Could you check a few things on this model? Use its own coordinates, in mm. Face numbers are marked on the shaded views. A direction names the side the tool comes from. Give positions to 0.01 mm unless a question says otherwise; leave off trailing zeros. Write each loop counter-clockwise with the first axis right and the second up, starting at its lowest first coordinate (ties: lowest second). Pieces come first, ordered by that corner, then holes. Notation, with made-up numbers: M 68,-15.5 L 72,-15.5 A23 ccw 72,16.5 Z; hole C -37.75,-9 d9. An arc over 180 degrees is marked long. Use one line per item in the form item = value.
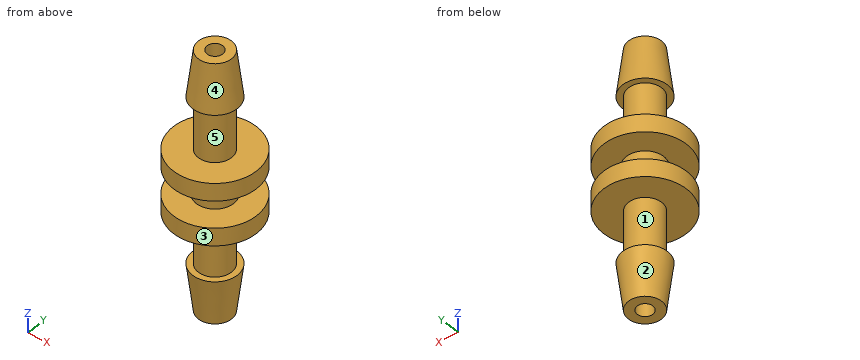
from build123d import *

# Parameters (mm, degrees)
SKETCH1_R           = 1.8
SKETCH1_R_2         = 0.75
BOSS_EXTRUDE1_DEPTH = 1.3
SKETCH2_R           = 4
SKETCH2_R_2         = 0.75
BOSS_EXTRUDE2_DEPTH = 1.7
SKETCH3_R           = 1.6
SKETCH3_R_2         = 0.75
BOSS_EXTRUDE3_DEPTH = 5


with BuildPart() as part:
    # Sketch1 → Boss-Extrude1 (new body)
    with BuildSketch(Plane.XY):
        Circle(SKETCH1_R)
        Circle(SKETCH1_R_2, mode=Mode.SUBTRACT)
    boss_extrude1 = extrude(amount=BOSS_EXTRUDE1_DEPTH)

    # Sketch2 → Boss-Extrude2 (add)
    with BuildSketch(Plane.XY.offset(1.3)):
        Circle(SKETCH2_R)
        Circle(SKETCH2_R_2, mode=Mode.SUBTRACT)
    boss_extrude2 = extrude(amount=BOSS_EXTRUDE2_DEPTH)

    # Sketch3 → Boss-Extrude3 (add)
    with BuildSketch(Plane.XY.offset(3)):
        Circle(SKETCH3_R)
        Circle(SKETCH3_R_2, mode=Mode.SUBTRACT)
    boss_extrude3 = extrude(amount=BOSS_EXTRUDE3_DEPTH)

    # Sketch5 → Revolve1 (revolve)
    with BuildSketch(Plane(origin=(0, 0, 0), x_dir=(1, 0, 0), z_dir=(0, 1, 0))):
        Polygon((0.75, -8), (0.75, -12.5), (1.6, -12.5), (2.15, -8), align=None)
    revolve1 = revolve(axis=Axis((0, 0, 0), (0, 0, 1)))

    # Mirror1: Boss-Extrude1, Boss-Extrude2, Boss-Extrude3, Revolve1 across plane
    add(boss_extrude1.mirror(Plane.XY))
    add(boss_extrude2.mirror(Plane.XY))
    add(boss_extrude3.mirror(Plane.XY))
    add(revolve1.mirror(Plane.XY))


solid = part.part
1) I want a section at D-D, the plane y = -3. Please give me the cut outline in (x, z), plus the area to 3 significant figures.
Checked values:
outline = M -2.65,-3 L 2.65,-3 L 2.65,-1.3 L -2.65,-1.3 Z; M -2.65,1.3 L 2.65,1.3 L 2.65,3 L -2.65,3 Z
area = 18.0 mm2
2) For the marked faces 4 and 5, which set-ups out of +Z, -Z, +X, -X, +Y, -Y let a thin tool reach every point of the face, with its end or its side?
Checked values:
face_4 = +Z
face_5 = none
3) I want a section at C-C, the plane z = -0.5. Please give me the cut outline in (x, y).
Checked values:
outline = C 0,0 d3.6; hole C 0,0 d1.5
4) Thinking about a two-plate mould opening in Z: for the marked faces 1, 2 and 3, which applies, released by +Z, released by -Z, zero draft, split by the parting line, or undercut?
Checked values:
face_1 = undercut
face_2 = released by -Z
face_3 = zero draft
5) For pin 1 Ø2 at (y, z) = (-3, 7) entering from -X; pin 2 Ø1.5 at (y, z) = (1.5, -2) entering from +X; pin 3 Ø2.5 at (x, y) = (-1, -1.5) entering from +Z; pin 4 Ø4 at (y, z) = (-2.5, 9.5) entering from +X, each with a flat end and sliding along its axis, tell me the tip position at first contact or that it passes through.
Checked values:
pin_1 = through
pin_2 = 3.93
pin_3 = 12.5
pin_4 = 1.95
6) If I drill on L1, parallel to Z at x = 0.25, y = 2.75; L2, parallel to Y at x = 0, z = 0; L3, parallel to Y at x = 0, z = -10.3, over which ranges is the centre line in solid material (lowest first)?
Checked values:
L1 = -3 to -1.3, 1.3 to 3
L2 = -1.8 to -0.75, 0.75 to 1.8
L3 = -1.87 to -0.75, 0.75 to 1.87
